Can you work these out from the model? Positions are in its coordinate system, mm. Coordinates: 2 decimals unless noted, no trailing zeros. Order: outer loops, then holes, each group sorted by start corner. A loop starts at its lowest first (then second) coordinate and runs counter-clockwise, first axis right, second up. Notation, with made-up numbers: (2.5, -12) - (57.5, -12) arc R21 ccw to (57.5, 8) - close; hole circle Ø3 at (-18, 69). An arc over 180 degrees is marked (long way). Use a Markdown table: item, result. Add a question column.
(1) For pin 1 Ø2 at (x, y) = (-48.5, 2.5) entering from -Z; pin 2 Ø4 at (x, z) = (-49, 58.7) entering from +Y; pin 3 Ø1.2 at (y, z) = (1, -137.5) entering from -X, each with a flat end and sliding along its axis, tell me the tip position at first contact or that it passes through.
(2) I want a section at B-B (y = 1.5). State how many separate pieces and enclosed holes the cut face has, and give its area (3 significant figures).
(3) I want a section at A-A (x = -49). List the corners of the cut face in (y, z) for me, and give its area (3 significant figures).
(4) If I drill on L1, parallel to X at y = 2.45, z = 48.62; L2, parallel to X at y = 3.1, z = 58.7; L3, parallel to X at y = 1.2, z = -149.95, over which ranges is the centre line in solid material (lowest first)? Write a range as [from, to].
(5) I want a section at D-D (z = -136). List the corners of the cut face in (x, y) for me.
(6) I want a section at C-C (x = 5). List the corners of the cut face in (y, z) for me.
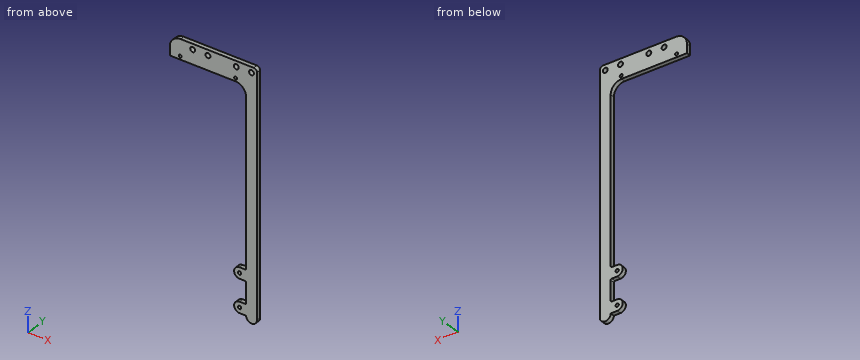
```python
from build123d import *

# Parameters (mm, degrees)
BOSS_EXTRUDE1_DEPTH = 4
SKETCH3_R           = 1.35
SKETCH3_R_2         = 2.25
BOSS_EXTRUDE3_DEPTH = 4
FILLET2_R           = 3
SKETCH6_R           = 1.5
BOSS_EXTRUDE5_DEPTH = 4
FILLET4_R           = 1
FILLET5_R           = 10


with BuildPart() as part:
    # Sketch1 → Boss-Extrude1 (new body)
    with BuildSketch(Plane(origin=(0, 0, 0), x_dir=(1, 0, 0), z_dir=(0, 1, 0))):
        with BuildLine():
            Line((0, 154.95), (0, 0))
            Line((0, 0), (10, 0))
            Line((10, 0), (10, 154.95))
            ThreePointArc((10, 154.95), (5, 159.95), (0, 154.95))
        make_face()
    extrude(amount=BOSS_EXTRUDE1_DEPTH)

    # Sketch3 → Boss-Extrude3 (add)
    with BuildSketch(Plane(origin=(0, 4, 0), x_dir=(1, 0, 0), z_dir=(0, 1, 0))):
        with BuildLine():
            Line((0, 0), (0, -45.7))
            Line((0, -45.7), (-70, -45.7))
            Line((-70, -45.7), (-70, -53.7))
            ThreePointArc((-70, -53.7), (-67.071067812, -60.771067812), (-60, -63.7))
            Line((-60, -63.7), (10, -63.7))
            Line((10, -63.7), (10, 0))
            Line((10, 0), (0, 0))
        make_face()
        with Locations((-60.4, -48.62)):
            Circle(SKETCH3_R, mode=Mode.SUBTRACT)
        with Locations((-49, -58.7)):
            Circle(SKETCH3_R_2, mode=Mode.SUBTRACT)
        with Locations((-35, -58.7)):
            Circle(SKETCH3_R_2, mode=Mode.SUBTRACT)
        with Locations((-9, -58.7)):
            Circle(SKETCH3_R_2, mode=Mode.SUBTRACT)
        with Locations((-9.6, -48.62)):
            Circle(SKETCH3_R, mode=Mode.SUBTRACT)
        with Locations((5, -58.7)):
            Circle(SKETCH3_R_2, mode=Mode.SUBTRACT)
    extrude(amount=-BOSS_EXTRUDE3_DEPTH)

    # Fillet2
    fillet2_edges = [part.edges().sort_by_distance(p)[0] for p in [
        (10, 2, 63.7),
    ]]
    fillet(fillet2_edges, radius=FILLET2_R)

    # Sketch6 → Boss-Extrude5 (add)
    with BuildSketch(Plane(origin=(0, 4, 0), x_dir=(1, 0, 0), z_dir=(0, 1, 0))):
        with BuildLine():
            Line((0, 154.95), (-6, 154.95))
            ThreePointArc((-6, 154.95), (-11, 149.95), (-6, 144.95))
            Line((-6, 144.95), (0, 144.95))
            Line((0, 144.95), (0, 154.95))
        make_face()
        with Locations((-6, 149.95)):
            Circle(SKETCH6_R, mode=Mode.SUBTRACT)
        with BuildLine():
            Line((0, 114.95), (0, 124.95))
            Line((0, 124.95), (-6, 124.95))
            ThreePointArc((-6, 124.95), (-11, 119.95), (-6, 114.95))
            Line((-6, 114.95), (0, 114.95))
        make_face()
        with Locations((-6, 119.95)):
            Circle(SKETCH6_R, mode=Mode.SUBTRACT)
    extrude(amount=-BOSS_EXTRUDE5_DEPTH)

    # Fillet4
    fillet4_edges = [part.edges().sort_by_distance(p)[0] for p in [
        (0, 2, -144.95),
        (0, 2, -124.95),
        (0, 2, -114.95),
    ]]
    fillet(fillet4_edges, radius=FILLET4_R)

    # Fillet5
    fillet5_edges = [part.edges().sort_by_distance(p)[0] for p in [
        (0, 2, 45.7),
    ]]
    fillet(fillet5_edges, radius=FILLET5_R)


solid = part.part
```
Answers follow:
| question | item | result |
|---|---|---|
| 1 | pin 1 | stops at z = 45.7 |
| 1 | pin 2 | passes through |
| 1 | pin 3 | stops at x = 0 |
| 2 | separate pieces | 1 |
| 2 | enclosed holes | 8 |
| 2 | area | 3,590 mm² |
| 3 | outline | (0, 45.7) - (4, 45.7) - (4, 56.45) - (0, 56.45) - close; (0, 60.95) - (4, 60.95) - (4, 63.7) - (0, 63.7) - close |
| 3 | area | 54.0 mm² |
| 4 | L1 | x = [-70, -61.75], [-59.05, -10.95], [-8.25, 10] |
| 4 | L2 | x = [-68.66, -51.25], [-46.75, -37.25], [-32.75, -11.25], [-6.75, 2.75], [7.25, 10] |
| 4 | L3 | x = [-11, -7.5], [-4.5, 10] |
| 5 | outline | (0, 0) - (10, 0) - (10, 4) - (0, 4) - close |
| 6 | outline | (0, -159.95) - (4, -159.95) - (4, 56.45) - (0, 56.45) - close; (0, 60.95) - (4, 60.95) - (4, 63.7) - (0, 63.7) - close |
